from build123d import *

# Parameters (mm, degrees)
SKETCH_1_W      = 100
SKETCH_1_H      = 80
SKETCH_1_R      = 1.6
EXTRUDE_1_DEPTH = 3


with BuildPart() as part:
    # 草图1 → 凸台-拉伸1 (new body)
    with BuildSketch(Plane(origin=(0, 0, 0), x_dir=(1, 0, 0), z_dir=(0, 1, 0))):
        Rectangle(SKETCH_1_W, SKETCH_1_H)
        with Locations(Location((-18, 22.242640687, 0), (0, 0, 270))):
            Circle(SKETCH_1_R, mode=Mode.SUBTRACT)
        with Locations(Location((18, 22.242640687, 0), (0, 0, 270))):
            Circle(SKETCH_1_R, mode=Mode.SUBTRACT)
        with Locations(Location((-18, -22.242640687, 0), (0, 0, 270))):
            Circle(SKETCH_1_R, mode=Mode.SUBTRACT)
        with Locations(Location((18, -22.242640687, 0), (0, 0, 270))):
            Circle(SKETCH_1_R, mode=Mode.SUBTRACT)
        with Locations(Location((-9, 21, 0), (0, 0, 270))):
            Circle(SKETCH_1_R, mode=Mode.SUBTRACT)
        with Locations(Location((9, 21, 0), (0, 0, 270))):
            Circle(SKETCH_1_R, mode=Mode.SUBTRACT)
        with Locations(Location((10, -21, 0), (0, 0, 270))):
            Circle(SKETCH_1_R, mode=Mode.SUBTRACT)
        with Locations(Location((-8, -21, 0), (0, 0, 270))):
            Circle(SKETCH_1_R, mode=Mode.SUBTRACT)
        with Locations(Location((-44.080756497, 30, 0), (0, 0, 270))):
            Circle(SKETCH_1_R, mode=Mode.SUBTRACT)
        with Locations(Location((44.080756497, 30, 0), (0, 0, 90))):
            Circle(SKETCH_1_R, mode=Mode.SUBTRACT)
        with Locations(Location((-44.080756497, -30, 0), (0, 0, 90))):
            Circle(SKETCH_1_R, mode=Mode.SUBTRACT)
        with Locations(Location((44.080756497, -30, 0), (0, 0, 270))):
            Circle(SKETCH_1_R, mode=Mode.SUBTRACT)
        Polygon((0, 5), (-4.330127019, 2.5), (-4.330127019, -2.5), (0, -5), (4.330127019, -2.5), (4.330127019, 2.5), align=None, mode=Mode.SUBTRACT)
        Polygon((5, -3), (0.669872981, -5.5), (0.669872981, -10.5), (5, -13), (9.330127019, -10.5), (9.330127019, -5.5), align=None, mode=Mode.SUBTRACT)
        Polygon((10, 5), (5.669872981, 2.5), (5.669872981, -2.5), (10, -5), (14.330127019, -2.5), (14.330127019, 2.5), align=None, mode=Mode.SUBTRACT)
        Polygon((20, 5), (15.669872981, 2.5), (15.669872981, -2.5), (20, -5), (24.330127019, -2.5), (24.330127019, 2.5), align=None, mode=Mode.SUBTRACT)
        Polygon((30, 5), (25.669872981, 2.5), (25.669872981, -2.5), (30, -5), (34.330127019, -2.5), (34.330127019, 2.5), align=None, mode=Mode.SUBTRACT)
        Polygon((40, 5), (35.669872981, 2.5), (35.669872981, -2.5), (40, -5), (44.330127019, -2.5), (44.330127019, 2.5), align=None, mode=Mode.SUBTRACT)
        Polygon((-44.330127019, 2.5), (-40, 5), (-35.669872981, 2.5), (-35.669872981, -2.5), (-40, -5), (-44.330127019, -2.5), align=None, mode=Mode.SUBTRACT)
        Polygon((-34.330127019, 2.5), (-30, 5), (-25.669872981, 2.5), (-25.669872981, -2.5), (-30, -5), (-34.330127019, -2.5), align=None, mode=Mode.SUBTRACT)
        Polygon((-24.330127019, 2.5), (-20, 5), (-15.669872981, 2.5), (-15.669872981, -2.5), (-20, -5), (-24.330127019, -2.5), align=None, mode=Mode.SUBTRACT)
        Polygon((-14.330127019, 2.5), (-10, 5), (-5.669872981, 2.5), (-5.669872981, -2.5), (-10, -5), (-14.330127019, -2.5), align=None, mode=Mode.SUBTRACT)
        Polygon((15, -3), (10.669872981, -5.5), (10.669872981, -10.5), (15, -13), (19.330127019, -10.5), (19.330127019, -5.5), align=None, mode=Mode.SUBTRACT)
        Polygon((25, -3), (20.669872981, -5.5), (20.669872981, -10.5), (25, -13), (29.330127019, -10.5), (29.330127019, -5.5), align=None, mode=Mode.SUBTRACT)
        Polygon((35, -3), (30.669872981, -5.5), (30.669872981, -10.5), (35, -13), (39.330127019, -10.5), (39.330127019, -5.5), align=None, mode=Mode.SUBTRACT)
        Polygon((45, -3), (40.669872981, -5.5), (40.669872981, -10.5), (45, -13), (49.330127019, -10.5), (49.330127019, -5.5), align=None, mode=Mode.SUBTRACT)
        Polygon((-49.330127019, -5.5), (-45, -3), (-40.669872981, -5.5), (-40.669872981, -10.5), (-45, -13), (-49.330127019, -10.5), align=None, mode=Mode.SUBTRACT)
        Polygon((-39.330127019, -5.5), (-35, -3), (-30.669872981, -5.5), (-30.669872981, -10.5), (-35, -13), (-39.330127019, -10.5), align=None, mode=Mode.SUBTRACT)
        Polygon((-29.330127019, -5.5), (-25, -3), (-20.669872981, -5.5), (-20.669872981, -10.5), (-25, -13), (-29.330127019, -10.5), align=None, mode=Mode.SUBTRACT)
        Polygon((-19.330127019, -5.5), (-15, -3), (-10.669872981, -5.5), (-10.669872981, -10.5), (-15, -13), (-19.330127019, -10.5), align=None, mode=Mode.SUBTRACT)
        Polygon((-9.330127019, -5.5), (-5, -3), (-0.669872981, -5.5), (-0.669872981, -10.5), (-5, -13), (-9.330127019, -10.5), align=None, mode=Mode.SUBTRACT)
        Polygon((49.330127019, 5.5), (45, 3), (40.669872981, 5.5), (40.669872981, 10.5), (45, 13), (49.330127019, 10.5), align=None, mode=Mode.SUBTRACT)
        Polygon((39.330127019, 5.5), (35, 3), (30.669872981, 5.5), (30.669872981, 10.5), (35, 13), (39.330127019, 10.5), align=None, mode=Mode.SUBTRACT)
        Polygon((29.330127019, 5.5), (25, 3), (20.669872981, 5.5), (20.669872981, 10.5), (25, 13), (29.330127019, 10.5), align=None, mode=Mode.SUBTRACT)
        Polygon((19.330127019, 5.5), (15, 3), (10.669872981, 5.5), (10.669872981, 10.5), (15, 13), (19.330127019, 10.5), align=None, mode=Mode.SUBTRACT)
        Polygon((9.330127019, 5.5), (5, 3), (0.669872981, 5.5), (0.669872981, 10.5), (5, 13), (9.330127019, 10.5), align=None, mode=Mode.SUBTRACT)
        Polygon((-9.330127019, 10.5), (-9.330127019, 5.5), (-5, 3), (-0.669872981, 5.5), (-0.669872981, 10.5), (-5, 13), align=None, mode=Mode.SUBTRACT)
        Polygon((-19.330127019, 10.5), (-19.330127019, 5.5), (-15, 3), (-10.669872981, 5.5), (-10.669872981, 10.5), (-15, 13), align=None, mode=Mode.SUBTRACT)
        Polygon((-29.330127019, 10.5), (-29.330127019, 5.5), (-25, 3), (-20.669872981, 5.5), (-20.669872981, 10.5), (-25, 13), align=None, mode=Mode.SUBTRACT)
        Polygon((-39.330127019, 10.5), (-39.330127019, 5.5), (-35, 3), (-30.669872981, 5.5), (-30.669872981, 10.5), (-35, 13), align=None, mode=Mode.SUBTRACT)
        Polygon((-49.330127019, 10.5), (-49.330127019, 5.5), (-45, 3), (-40.669872981, 5.5), (-40.669872981, 10.5), (-45, 13), align=None, mode=Mode.SUBTRACT)
    extrude(amount=EXTRUDE_1_DEPTH)


solid = part.part
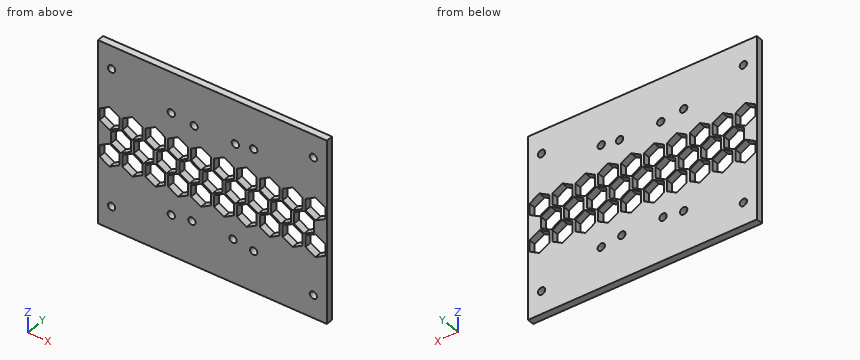
The listing builds one solid part. Answer for the finished solid, in the listing's coordinates (mm). Round coordinates to 2 decimals unless told otherwise and drop trailing zeros. Loops run counter-clockwise (first coordinate to the right, second up) from the corner with the lowest first, then second, coordinate; pieces in that order, holes last. Notation, with made-up numbers: M 68,61 L 99,61 A20 cw 99,83 Z; hole C 16.25,35 d2. An arc over 180 degrees is marked long. Return JSON: item names as keys, results as strings.
Q1. Find section B-B, the plane x = 18. Determine the outline of the cut face in (y, z), plus the area to 3 significant figures.
Results list:
{"outline": "M 0,-40 L 3,-40 L 3,-23.84 L 0,-23.84 Z; M 0,-20.64 L 3,-20.64 L 3,-11.27 L 0,-11.27 Z; M 0,-4.73 L 3,-4.73 L 3,-3.85 L 0,-3.85 Z; M 0,3.85 L 3,3.85 L 3,4.73 L 0,4.73 Z; M 0,11.27 L 3,11.27 L 3,20.64 L 0,20.64 Z; M 0,23.84 L 3,23.84 L 3,40 L 0,40 Z", "area": "159 mm2"}
Q2. Find section A-A, the plane z = -30. Determine the outline of the cut face in (x, y).
Results list:
{"outline": "M -50,0 L -45.68,0 L -45.68,3 L -50,3 Z; M -42.48,0 L 42.48,0 L 42.48,3 L -42.48,3 Z; M 45.68,0 L 50,0 L 50,3 L 45.68,3 Z"}
Q3. Find the intervals of material crossed by line 1 along X through (y, z) = (0.8, 30); line 2 along Z through (x, y) = (-14.5, 2.6); line 3 along Z through (x, y) = (35, 1.8), in increasing order. Write a range as from..to.
Results list:
{"line 1": "x = -50..-45.68, -42.48..42.48, 45.68..50", "line 2": "z = -40..-12.71, -3.29..3.29, 12.71..40", "line 3": "z = -40..-13, -3..3, 13..40"}
Q4. This flat-tipped pin is pushed along its axis until it touches: pin 1 Ø2.5 at (x, z) = (-9, -21) entering from -Y. Where does it stop, or does it pass through?
Results list:
{"pin 1": "passes through"}
Q5. Find section C-C, the plane y = 0.6. State how many separate pieces and enclosed holes the cut face has, plus the area to 3 significant figures.
Results list:
{"separate pieces": "1", "enclosed holes": "41", "area": "6,020 mm2"}
